Read the model definition and answer for the solid it produces. Units are mm, in the model's axes. A direction names the side the tool comes from. Give positions to 0.01 mm unless a question says otherwise; leave off trailing zeros. Order: outer loops, then holes, each group sorted by start corner. A loop starts at its lowest first (then second) coordinate and runs counter-clockwise, first axis right, second up. Notation, with made-up numbers: (10, 33) - (55, 33) arc R35 ccw to (55, 68) - close; hole circle Ø5 at (67.25, 84.5). An arc over 180 degrees is marked (long way). Return JSON: item names as keys, results as strings.
```python
from build123d import *

# Parameters (mm, degrees)
SKETCH_1_W                    = 25
SKETCH_1_H                    = 12
SKETCH_1_W_2                  = 21
SKETCH_1_H_2                  = 8
EXTRUDE_1_DEPTH               = 56
CUT_EXTRUDE_1_REACH           = 14
SKETCH_2_R                    = 9
HOLE_WIZARD_4_40_1_AT_2_COUNT = 2
HOLE_WIZARD_4_40_1_AT_2_PITCH = 48.7
HOLE_WIZARD_4_40_1_AT_3_COUNT = 2
HOLE_WIZARD_4_40_1_AT_3_PITCH = 49.716093974
HOLE_WIZARD_4_40_1_AT_4_COUNT = 2
HOLE_WIZARD_4_40_1_AT_4_PITCH = 10
CUT_EXTRUDE_2_DEPTH           = 6
CUT_EXTRUDE_4_DEPTH           = 1
SKETCH_9_W                    = 25
SKETCH_9_H                    = 19
CUT_EXTRUDE_7_DEPTH           = 10
CUT_EXTRUDE_8_REACH           = 27
CUT_EXTRUDE_9_DEPTH           = 3
SKETCH_15_W                   = 3
SKETCH_15_H                   = 2
CUT_EXTRUDE_10_DEPTH          = 26
HOLE_WIZARD_M31_D             = 3.6
HOLE_WIZARD_M31_CSINK_D       = 5.5
HOLE_WIZARD_M31_CSINK_ANGLE   = 90
CUT_EXTRUDE_11_DEPTH          = 0.7


with BuildPart() as part:
    # Sketch 1 → Extrude 1 (new body)
    with BuildSketch(Plane.XY):
        Rectangle(SKETCH_1_W, SKETCH_1_H)
        Rectangle(SKETCH_1_W_2, SKETCH_1_H_2, mode=Mode.SUBTRACT)
    extrude(amount=EXTRUDE_1_DEPTH)

    # Sketch 2 → Cut-Extrude 1 (cut, up to next)
    with BuildSketch(Plane(origin=(0, 6, 0), x_dir=(1, 0, 0), z_dir=(0, 1, 0)), mode=Mode.PRIVATE) as cut_extrude_1_sk1:
        with Locations((0, -17.5)):
            Circle(SKETCH_2_R)
    cut_extrude_1_tool1 = extrude(cut_extrude_1_sk1.sketch, amount=-CUT_EXTRUDE_1_REACH, mode=Mode.PRIVATE) & part.part
    add(cut_extrude_1_tool1.solids().sort_by_distance((0, 6, 17.5))[0], mode=Mode.SUBTRACT)

    # Sketch 3 → Hole Wizard 4-40 - 1 (revolve, cut)
    with BuildSketch(Plane(origin=(5, -6, 52.2), x_dir=(0, 0, -1), z_dir=(1, 0, 0))):
        Polygon((0, 0), (0, 2), (1.6764, 2), (1.4224, 1.822147285), (1.4224, 0.177852715), (1.6764, 0), align=None)
    hole_wizard_4_40_1 = revolve(axis=Axis((5, -12.35, 52.2), (0, 1, 0)), mode=Mode.SUBTRACT)

    # Hole Wizard 4-40 - 1 at 2: Hole Wizard 4-40 - 1 ×2
    with Locations(*[(0, 0, -i * HOLE_WIZARD_4_40_1_AT_2_PITCH) for i in range(1, HOLE_WIZARD_4_40_1_AT_2_COUNT)]):
        add(hole_wizard_4_40_1, mode=Mode.SUBTRACT)

    # Hole Wizard 4-40 - 1 at 3: Hole Wizard 4-40 - 1 ×2
    with Locations(*[Vector(-0.201142109, 0, -0.979562072) * (i * HOLE_WIZARD_4_40_1_AT_3_PITCH) for i in range(1, HOLE_WIZARD_4_40_1_AT_3_COUNT)]):
        add(hole_wizard_4_40_1, mode=Mode.SUBTRACT)

    # Hole Wizard 4-40 - 1 at 4: Hole Wizard 4-40 - 1 ×2
    with Locations(*[(-i * HOLE_WIZARD_4_40_1_AT_4_PITCH, 0, 0) for i in range(1, HOLE_WIZARD_4_40_1_AT_4_COUNT)]):
        add(hole_wizard_4_40_1, mode=Mode.SUBTRACT)

    # Sketch 5 → Cut-Extrude 2 (cut)
    with BuildSketch(Plane.XZ.offset(6)):
        with BuildLine():
            Line((-12.5, 23.7), (-12.5, 11.3))
            Line((-12.5, 11.3), (0, 11.3))
            ThreePointArc((0, 11.3), (6.2, 17.5), (0, 23.7))
            Line((0, 23.7), (-12.5, 23.7))
        make_face()
    extrude(amount=-CUT_EXTRUDE_2_DEPTH, mode=Mode.SUBTRACT)

    # Sketch 8 → Cut-Extrude 4 (cut)
    with BuildSketch(Plane.ZY.offset(12.5)):
        with BuildLine():
            Line((9.3, -6), (9.3, -2))
            ThreePointArc((9.3, -2), (10.178679656, 0.121320344), (12.3, 1))
            Line((12.3, 1), (22.3, 1))
            ThreePointArc((22.3, 1), (24.421320344, 0.121320344), (25.3, -2))
            Line((25.3, -2), (25.3, -6))
            Line((25.3, -6), (9.3, -6))
        make_face()
    extrude(amount=-CUT_EXTRUDE_4_DEPTH, mode=Mode.SUBTRACT)

    # Sketch 9 → Cut-Extrude 7 (cut)
    with BuildSketch(Plane(origin=(0, 6, 0), x_dir=(1, 0, 0), z_dir=(0, 1, 0))):
        with Locations((0, -46.5)):
            Rectangle(SKETCH_9_W, SKETCH_9_H)
    extrude(amount=-CUT_EXTRUDE_7_DEPTH, mode=Mode.SUBTRACT)

    # Sketch 13 → Cut-Extrude 8 (cut, up to next)
    with BuildSketch(Plane(origin=(12.5, 0, 0), x_dir=(0, 0, -1), z_dir=(1, 0, 0)), mode=Mode.PRIVATE) as cut_extrude_8_sk1:
        with BuildLine():
            Line((-22.5, 3), (-12.5, 3))
            ThreePointArc((-12.5, 3), (-9.5, 0), (-12.5, -3))
            Line((-12.5, -3), (-22.5, -3))
            ThreePointArc((-22.5, -3), (-25.5, 0), (-22.5, 3))
        make_face()
    cut_extrude_8_tool1 = extrude(cut_extrude_8_sk1.sketch, amount=-CUT_EXTRUDE_8_REACH, mode=Mode.PRIVATE) & part.part
    add(cut_extrude_8_tool1.solids().sort_by_distance((12.5, 0, 17.5))[0], mode=Mode.SUBTRACT)

    # Sketch 14 → Cut-Extrude 9 (cut)
    with BuildSketch(Plane(origin=(0, 6, 0), x_dir=(1, 0, 0), z_dir=(0, 1, 0))):
        with BuildLine():
            Line((-4.124545619, -33.5), (0, -33.5))
            ThreePointArc((0, -33.5), (2.958039892, -34.468871126), (4.769696007, -37))
            Line((4.769696007, -37), (-12.5, -37))
            Line((-12.5, -37), (-12.5, -15.538780117))
            Line((-12.5, -15.538780117), (-4.124545619, -33.5))
        make_face()
    extrude(amount=-CUT_EXTRUDE_9_DEPTH, mode=Mode.SUBTRACT)

    # Sketch 15 → Cut-Extrude 10 (cut, through all)
    with BuildSketch(Plane.ZY.offset(12.5)):
        with Locations((35.5, -3)):
            Rectangle(SKETCH_15_W, SKETCH_15_H)
        with Locations((1.5, -1)):
            Rectangle(SKETCH_15_W, SKETCH_15_H)
    extrude(amount=-CUT_EXTRUDE_10_DEPTH, mode=Mode.SUBTRACT)

    # Hole Wizard M31 (through all)
    with Locations(Plane.XZ.offset(6)):
        with Locations((0, 40)):
            CounterSinkHole(HOLE_WIZARD_M31_D / 2, HOLE_WIZARD_M31_CSINK_D / 2, counter_sink_angle=HOLE_WIZARD_M31_CSINK_ANGLE)

    # Sketch 18 → Cut-Extrude 11 (cut)
    with BuildSketch(Plane(origin=(0, -4, 0), x_dir=(1, 0, 0), z_dir=(0, 1, 0))):
        with BuildLine():
            Line((-2, -38), (2, -38))
            ThreePointArc((2, -38), (4, -40), (2, -42))
            Line((2, -42), (-2, -42))
            ThreePointArc((-2, -42), (-4, -40), (-2, -38))
        make_face()
    extrude(amount=-CUT_EXTRUDE_11_DEPTH, mode=Mode.SUBTRACT)


solid = part.part
```
Q1. A cutting plane is placed at B-B (y = 5). Write down the section's boundary in (x, z).
Values:
{"outline": "(-12.5, 0) - (12.5, 0) - (12.5, 37) - (4.77, 37) arc R5 cw to (0, 33.5) - (-4.12, 33.5) - (-12.5, 15.54) - close; hole circle Ø18 at (0, 17.5)"}
Q2. A cutting plane is placed at D-D (x = -9.5). Write down the section's boundary in (y, z), and give its area (3 significant figures).
Values:
{"outline": "(-6, 0) - (-4, 0) - (-4, 11.3) - (-6, 11.3) - close; (-6, 23.7) - (-4, 23.7) - (-4, 56) - (-6, 56) - close; (4, 0) - (6, 0) - (6, 21.97) - (4, 21.97) - close", "area": "131 mm²"}
Q3. A cutting plane is placed at A-A (z = 40). Write down the section's boundary in (x, y), and give its area (3 significant figures).
Values:
{"outline": "(-12.5, -6) - (-2.75, -6) - (-1.8, -5.05) - (-1.8, -4.7) - (-4, -4.7) - (-4, -4) - (-12.5, -4) - close; (1.8, -5.05) - (2.75, -6) - (12.5, -6) - (12.5, -4) - (4, -4) - (4, -4.7) - (1.8, -4.7) - close", "area": "38.8 mm²"}
Q4. Given pin 1 (2 mm diameter, centred on x = -12, z = 30.5, fed in from +Y); pin 2 (5 mm diameter, centred on x = -3, y = -2, fed in from +Z); pin 3 (3 mm diameter, centred on x = 1, y = -1.5, fed in from -Z); pin 4 (1 mm diameter, centred on x = -11.5, y = 1.5, fed in from +Z), each flat-ended and moving along its own axis, determine where each tip first touches the part or whether it passes through.
Values:
{"pin 1": "stops at y = 3", "pin 2": "stops at z = 56", "pin 3": "passes through", "pin 4": "stops at z = 37"}
Q5. A cutting plane is placed at C-C (z = 52.2). Write down the section's boundary in (x, y), and give its area (3 significant figures).
Values:
{"outline": "(-12.5, -6) - (-6.68, -6) - (-6.42, -5.82) - (-6.42, -4.18) - (-6.68, -4) - (-12.5, -4) - close; (-3.58, -5.82) - (-3.32, -6) - (3.32, -6) - (3.58, -5.82) - (3.58, -4.18) - (3.32, -4) - (-3.32, -4) - (-3.58, -4.18) - close; (6.42, -5.82) - (6.68, -6) - (12.5, -6) - (12.5, -4) - (6.68, -4) - (6.42, -4.18) - close", "area": "38.4 mm²"}
Q6. For faces 4 (the flat face through (11, -2, 1)), 5 (the flat face through (7, 4, 10)), 6 (the flat face through (12, -3, 17)), 7 (the flat face through (-7.1, -4.4, 11.3)), determine the directions among +Z, -Z, +X, -X, +Y, -Y from which every point of the face is accessible in a straight line to the end or side of a thin tool.
Values:
{"face 4": "-Z, +X, -X", "face 5": "+Z, -Z", "face 6": "+X, -X", "face 7": "-X, -Y"}
Q7. Consider L1, parallel to X at y = -4.6, z = 52.2; L2, parallel to Z at x = 0, y = 5.55; L3, parallel to Y at x = 1, z = 3. Determine where each line is inside the solid, lowest interval first.
Values:
{"L1": "x = -12.5 to -6.42, -3.58 to 3.58, 6.42 to 12.5", "L2": "z = 0 to 8.5, 26.5 to 33.5", "L3": "y = -6 to -4, 4 to 6"}
Q8. Determine the mould class of faces 1 (the flat face through (2, -4.7, 40)), 2 (the flat face through (-12, 1, 37)), 3 (the flat face through (12, 3, 18)) for opening direction Y: released by +Y, released by -Y, zero draft, split by the parting line, or undercut.
Values:
{"face 1": "released by +Y", "face 2": "zero draft", "face 3": "undercut"}
